Could you check a few things on this model? Use its own coordinates, in mm. Face numbers are marked on the shaded views. A direction names the side the tool comes from. Round coordinates to 2 decimals unless told otherwise and drop trailing zeros. Loops run counter-clockwise (first coordinate to the right, second up) from the corner with the lowest first, then second, coordinate; pieces in that order, holes last. Notation, with made-up numbers: (-16.5, -12.75) -> (29.5, -12.75) arc R7 cw to (29.5, -0.75) -> close; hole circle Ø9 at (-29, 26.5). An arc over 180 degrees is marked (long way). Put each result on its own line as item: value. Start each with the question number.
1. Imagine slicing it at A-A, the plane z = 10. Please give me the cut outline in (x, y).
2. If we mould it in two halves opening along Y, with no side actions, what happens to the marked faces 4, 5 and 6? For each: pulls with the +Y half, pulls with the -Y half, needs draft (parallel to the pull), parting line crosses it, or undercut.
3. I need wall thicknesses on line 1 (Z direction, x = 6, y = 11); line 2 (Y direction, x = -19, z = -10); line 3 (X direction, y = 14.25, z = 6.5). Which ranges of each line are inside material? Lowest first, please. Write a range as [from, to].
4. Imagine slicing it at C-C, the plane x = 5. Please give me the cut outline in (y, z).
5. Which directions (+Z, -Z, +X, -X, +Y, -Y) give clear straight access to the entire face, cutting with the end or side of a thin tool? Please do the marked faces 1, 2 and 3.
6. Imagine slicing it at D-D, the plane y = 5.5. Please give me the cut outline in (x, z), and give its area (3 significant figures).
7. Imagine slicing it at B-B, the plane y = 10. Count the separate pieces of the cut face and the enclosed holes in it, and give its area (3 significant figures).
8. I'm going to push flat-ended pins straight in: P1, Ø1.5, axis at x = -23.5, z = 10, coming from the +Y side; P2, Ø1, axis at x = 7.5, y = 6.5, coming from the -Z side; P3, Ø3, axis at y = 8, z = 9, coming from the -X side. Where does each tip first touch, or does it pass through?
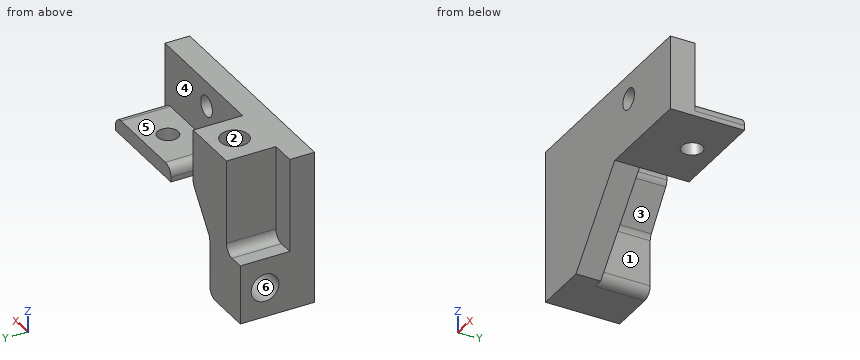
```python
from build123d import *

# Parameters (mm, degrees)
ESQUISSE1_R             = 2.1
BOSS_EXTRU_1_DEPTH      = 5
ESQUISSE2_W             = 20
ESQUISSE2_H             = 3
BOSS_EXTRU_2_DEPTH      = 10
ESQUISSE3_R             = 2.8
ENL_V_MAT_EXTRU_1_DEPTH = 9.1
ESQUISSE4_R             = 2.1
ENL_V_MAT_EXTRU_2_DEPTH = 9.1
CONG_2_R                = 2
ESQUISSE5_R             = 2.8
ENL_V_MAT_EXTRU_3_DEPTH = 9.1


with BuildPart() as part:
    # Esquisse1 → Boss.-Extru.1 (new body)
    with BuildSketch(Plane(origin=(0, 0, 0), x_dir=(1, 0, 0), z_dir=(0, 1, 0))):
        Polygon((20, 0), (20, -15), (-20, -15), (-25, -15), (-25, 16), (-14, 16), (0, 0), align=None)
        with Locations(Location((5, -10, 0), (0, 0, 270))):
            Circle(ESQUISSE1_R, mode=Mode.SUBTRACT)
    extrude(amount=BOSS_EXTRU_1_DEPTH)

    # Esquisse2 → Boss.-Extru.2 (add)
    with BuildSketch(Plane(origin=(0, 5, 0), x_dir=(1, 0, 0), z_dir=(0, 1, 0))):
        with Locations((10, -1.5)):
            Rectangle(ESQUISSE2_W, ESQUISSE2_H)
        Polygon((-14, 4), (-14, 16), (-25, 16), (-25, 4), (-20, 4), (-20, -15), (-8, -15), (-8, -4), align=None)
    extrude(amount=BOSS_EXTRU_2_DEPTH)

    # Esquisse3 → Enlèv. mat.-Extru.1 (cut)
    with BuildSketch(Plane.XY.offset(15)):
        with Locations((-14, 10)):
            Circle(ESQUISSE3_R)
    extrude(amount=-ENL_V_MAT_EXTRU_1_DEPTH, mode=Mode.SUBTRACT)

    # Esquisse4 → Enlèv. mat.-Extru.2 (cut)
    with BuildSketch(Plane.XY.offset(3)):
        with Locations((10, 10)):
            Circle(ESQUISSE4_R)
    extrude(amount=-ENL_V_MAT_EXTRU_2_DEPTH, mode=Mode.SUBTRACT)

    # Congé2
    cong_2_edges = [part.edges().sort_by_distance(p)[0] for p in [
        (0, 10, 3),
        (20, 10, 3),
        (-20, 10, -4),
        (-8, 10, 4),
        (-14, 10, -4),
        (-14, 10, -16),
    ]]
    fillet(cong_2_edges, radius=CONG_2_R)

    # Esquisse5 → Enlèv. mat.-Extru.3 (cut)
    with BuildSketch(Plane.ZY.offset(25)):
        with Locations((-10, 10)):
            Circle(ESQUISSE5_R)
    extrude(amount=-ENL_V_MAT_EXTRU_3_DEPTH, mode=Mode.SUBTRACT)


solid = part.part
```
Entries:
1. outline: (-25, 0) -> (2.9, 0) -> (2.9, 5) -> (-8, 5) -> (-8, 15) -> (-20, 15) -> (-20, 5) -> (-25, 5) -> close; (7.1, 0) -> (20, 0) -> (20, 5) -> (7.1, 5) -> close; hole circle Ø5.6 at (-14, 10)
2. face 4: pulls with the +Y half
2. face 5: needs draft
2. face 6: undercut
3. line 1: [0, 3]
3. line 2: [0, 7.2], [12.8, 15]
3. line 3: [-20, -8]
4. outline: (0, 0) -> (15, 0) -> (15, 3) -> (5, 3) -> (5, 7.9) -> (0, 7.9) -> close; (0, 12.1) -> (5, 12.1) -> (5, 15) -> (0, 15) -> close
5. face 1: -Z, +X, +Y
5. face 2: +Z
5. face 3: -Z, +Y
6. outline: (-25, -16) -> (-16, -16) arc R2 ccw to (-14, -14) -> (-14, -4.67) arc R2 cw to (-13.6, -3.47) -> (-8.4, 3.47) arc R2 ccw to (-8, 4.67) -> (-8, 15) -> (-20, 15) -> (-20, -2) arc R2 cw to (-22, -4) -> (-25, -4) -> close; (0, 0) -> (20, 0) -> (20, 1) arc R2 ccw to (18, 3) -> (2, 3) arc R2 ccw to (0, 1) -> close
6. area: 394 mm^2
7. separate pieces: 3
7. enclosed holes: 0
7. area: 280 mm^2
8. P1: y = 5
8. P2: z = 0
8. P3: x = -20
